Drawing for the job (mm, zero at the part's lowest x, y, z). A direction names the side the tool comes from. Round coordinates to 2 decimals unless told otherwise and drop trailing zeros. Write each loop counter-clockwise with the first axis right and the second up, starting at its lowest first coordinate (ties: lowest second). Pieces come first, ordered by that corner, then holes.
Item 1: Drop flat-ended pins along their axis: pin 1 Ø1 at (x, z) = (70.5, 23.5) entering from +Y; pin 2 Ø8 at (x, y) = (56, 14) entering from -Z; pin 3 Ø6.5 at (x, z) = (42, 14.5) entering from -Y. Give the stop position or say it passes through.
Item 2: Band-saw the part on C-C, the plane z = 7.5. Write the cut outline in (x, y).
Item 3: 3-axis set-ups, long thin cutter, end or side, ignore diameter. For the marked faces 1, 2 and 3: which of +Z, -Z, +X, -X, +Y, -Y reach the whole face in a straight line?
Item 4: Band-saw the part on A-A, the plane x = 41.5. Write the cut outline in (y, z).
Item 5: Wall check: probe 1 along Z at (x, y) = (13, 19.5); probe 2 along Y at (x, z) = (45, 29.5). Give the ranges that are in metal, low to high.
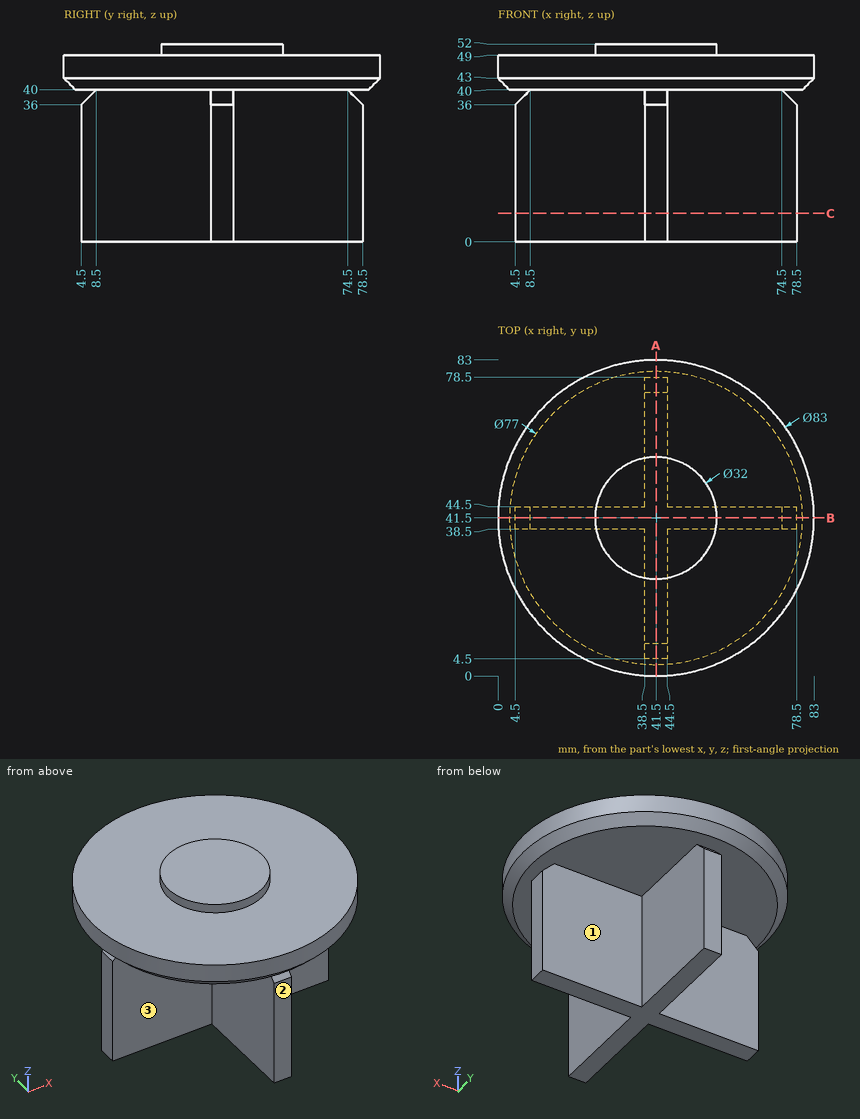
Results:
1. pin 1: stops at y = 44.5
1. pin 2: stops at z = 40
1. pin 3: stops at y = 4.5
2. outline: (4.5, 38.5) - (38.5, 38.5) - (38.5, 4.5) - (44.5, 4.5) - (44.5, 38.5) - (78.5, 38.5) - (78.5, 44.5) - (44.5, 44.5) - (44.5, 78.5) - (38.5, 78.5) - (38.5, 44.5) - (4.5, 44.5) - close
3. face 1: -Z, +X, +Y
3. face 2: -Z, +X, -X, -Y
3. face 3: -Z, -X, -Y
4. outline: (0, 43) - (3, 40) - (8.5, 40) - (4.5, 36) - (4.5, 0) - (78.5, 0) - (78.5, 36) - (74.5, 40) - (80, 40) - (83, 43) - (83, 49) - (57.5, 49) - (57.5, 52) - (25.5, 52) - (25.5, 49) - (0, 49) - close
5. probe 1: z = 40 to 49
5. probe 2: y = 38.5 to 44.5
